from build123d import *

# Parameters (mm, degrees)
F0_R     = 26.543977
F0_R_2   = 8.89
F1_DEPTH = 25.4
F3_DEPTH = 50.8
F4_R     = 26.543977
F5_DEPTH = 5.08


with BuildPart() as f1:
    # F0 (on Top) → F1 (new body)
    with BuildSketch(Plane.XY):
        Circle(F0_R)
        Circle(F0_R_2, mode=Mode.SUBTRACT)
    extrude(amount=F1_DEPTH)

    # F2 (on Right) → F3 (cut)
    with BuildSketch(Plane.YZ):
        with BuildLine():
            Line((-12.7, 17.921465), (-12.7, 0))
            Line((-12.7, 0), (12.7, 0))
            Line((12.7, 0), (12.7, 17.921465))
            ThreePointArc((12.7, 17.921465), (0, 22.035668), (-12.7, 17.921465))
        make_face()
    extrude(amount=-F3_DEPTH, mode=Mode.SUBTRACT)

    # F4 (on face) → F5 (join)
    with BuildSketch(Plane(origin=(0, 0, 0), x_dir=(1, 0, 0), z_dir=(0, 0, -1))):
        Circle(F4_R)
    extrude(amount=F5_DEPTH)


solid = f1.part
Work out the finished part from the listing and answer in its coordinate system (mm). A direction names the side the tool comes from. Round coordinates to 2 decimals unless told otherwise and drop trailing zeros. Write each loop counter-clockwise with the first axis right and the second up, starting at its lowest first coordinate (ties: lowest second). Pieces come first, ordered by that corner, then holes.
1) A tool of negligible diameter and unlimited length cuts with its end or side. For faces 4 (the cylindrical face through (8.48, 2.67, 15.34)), 5 (the flat face through (-11, 12.7, 9)), 6 (the cylindrical face through (24.52, 10.17, 10.37)), from which of +Z, -Z, +X, -X, +Y, -Y can it reach the whole face along a straight path? Write none if from no direction.
2) A cutting plane is placed at C-C (z = 5). Give the vertices of the cut face in (x, y), plus the area to 3 significant figures.
3) The mould has two halves that part along Z. Classify faces 1 (the flat face through (0, 0, -5.08)), 2 (the flat face through (11, 0, 25.4)), 3 (the flat face through (0, 11, 10)): pulls with the +Z half, pulls with the -Z half, needs draft (parallel to the pull), parting line crosses it, or undercut.
4) A cutting plane is placed at A-A (y = 0). Give the vertices of the cut face in (x, z).
5) Straight lines are drawn through the part: line 1 (Z direction, x = -2, y = 4); line 2 (X direction, y = 0, z = 8.25); line 3 (Z direction, x = -9.5, y = -2). For each, find the intervals that lie inside material, in ascending order.
6) A cutting plane is placed at D-D (x = -2). Give the vertices of the cut face in (y, z), plus the area to 3 significant figures.
7) A cutting plane is placed at B-B (x = -10.5). Give the vertices of the cut face in (y, z).
8) Given pin 1 Ø10 at (y, z) = (-5, 0.5) entering from +X; pin 2 Ø6 at (x, z) = (-17, -0.5) entering from -Y; pin 3 Ø12 at (x, z) = (6, 1) entering from -Y; pin 4 Ø1.9 at (y, z) = (11.5, 14.5) entering from -X, each flat-ended and moving along its own axis, determine where each tip first touches the part or whether it passes through.
Completed:
1. face 4: +Z
1. face 5: -X
1. face 6: +Z, -Z
2. outline: (-23.31, -12.7) arc R26.54 ccw (long way) to (-23.31, 12.7) - (0, 12.7) - (0, 8.89) arc R8.89 cw to (0, -8.89) - (0, -12.7) - close
2. area: 1,440 mm2
3. face 1: pulls with the -Z half
3. face 2: pulls with the +Z half
3. face 3: undercut
4. outline: (-26.54, -5.08) - (26.54, -5.08) - (26.54, 25.4) - (8.89, 25.4) - (8.89, 0) - (-26.54, 0) - close; (-26.54, 22.04) - (-8.89, 22.04) - (-8.89, 25.4) - (-26.54, 25.4) - close
5. line 1: z = -5.08 to 0
5. line 2: x = 8.89 to 26.54
5. line 3: z = -5.08 to 0, 21.94 to 25.4
6. outline: (-26.47, -5.08) - (26.47, -5.08) - (26.47, 25.4) - (8.66, 25.4) - (8.66, 20.23) arc R21.66 cw to (12.7, 17.92) - (12.7, 0) - (-12.7, 0) - (-12.7, 17.92) arc R21.66 cw to (-8.66, 20.23) - (-8.66, 25.4) - (-26.47, 25.4) - close
6. area: 1,020 mm2
7. outline: (-24.38, -5.08) - (24.38, -5.08) - (24.38, 25.4) - (-24.38, 25.4) - close; hole (-12.7, 0) - (12.7, 0) - (12.7, 17.92) arc R21.66 ccw to (-12.7, 17.92) - close
8. pin 1: stops at x = 26.54
8. pin 2: stops at y = -22.55
8. pin 3: stops at y = -26.54
8. pin 4: stops at x = 0
